Part model, mm, in its own coordinate system. Face numbers are marked on the shaded views. A direction names the side the tool comes from. Give positions to 0.01 mm unless a question says otherwise; leave off trailing zeros. Write each loop counter-clockwise with the first axis right and the second up, starting at its lowest first coordinate (ties: lowest second). Pieces come first, ordered by that corner, then holes.
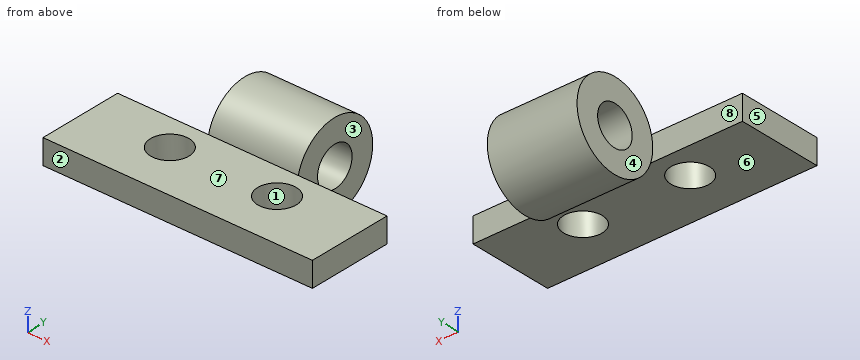
from build123d import *

# Parameters (mm, degrees)
SKETCH1_W           = 24.892
SKETCH1_H           = 7.874
BOSS_EXTRUDE1_DEPTH = 2.286
SKETCH4_R           = 4
BOSS_EXTRUDE3_DEPTH = 16.58
SKETCH5_R           = 1.825
CUT_EXTRUDE2_DEPTH  = 16.58
CUT_EXTRUDE3_DEPTH  = 8.29
SKETCH8_R           = 1.778
CUT_EXTRUDE4_DEPTH  = 8.29
SKETCH9_W           = 2.190957137
SKETCH9_H           = 1.309901185
SKETCH9_W_2         = 1.781735984
SKETCH9_H_2         = 0.803323297
CUT_EXTRUDE5_DEPTH  = 8.29


with BuildPart() as part:
    # Sketch1 → Boss-Extrude1 (new body)
    with BuildSketch(Plane.XY):
        with Locations((-11.83196875, 3.65678125)):
            Rectangle(SKETCH1_W, SKETCH1_H)
    extrude(amount=BOSS_EXTRUDE1_DEPTH)

    # Sketch4 → Boss-Extrude3 (add)
    with BuildSketch(Plane.ZY.offset(24.27796875)):
        with Locations((1.143, 11.58378125)):
            Circle(SKETCH4_R)
    extrude(amount=-BOSS_EXTRUDE3_DEPTH)

    # Sketch5 → Cut-Extrude2 (cut)
    with BuildSketch(Plane.ZY.offset(24.27796875)):
        with Locations((1.143, 11.58378125)):
            Circle(SKETCH5_R)
    extrude(amount=-CUT_EXTRUDE2_DEPTH, mode=Mode.SUBTRACT)

    # Sketch7 → Cut-Extrude3 (cut)
    with BuildSketch(Plane.ZY.offset(24.27796875)):
        Polygon((0.43016706, 7.59378125), (-5.580589686, 7.59378125), (-5.580589686, 19.623956734), (9.570834238, 19.623956734), (9.570834238, 7.59378125), align=None)
    extrude(amount=-CUT_EXTRUDE3_DEPTH, mode=Mode.SUBTRACT)

    # Sketch8 → Cut-Extrude4 (cut)
    with BuildSketch(Plane(origin=(0, 0, 0), x_dir=(-1, 0, 0), z_dir=(0, 0, -1))):
        with Locations((6.87896875, 4.54578125)):
            Circle(SKETCH8_R)
        with Locations((16.78496875, 4.54578125)):
            Circle(SKETCH8_R)
    extrude(amount=-CUT_EXTRUDE4_DEPTH, mode=Mode.SUBTRACT)

    # Sketch9 → Cut-Extrude5 (cut)
    with BuildSketch(Plane.ZY.offset(24.27796875)):
        with Locations((3.381478569, 7.915515048)):
            Rectangle(SKETCH9_W, SKETCH9_H)
        with Locations((-0.890867992, 7.662226104)):
            Rectangle(SKETCH9_W_2, SKETCH9_H_2)
    extrude(amount=-CUT_EXTRUDE5_DEPTH, mode=Mode.SUBTRACT)


solid = part.part
1) 3-axis set-ups, long thin cutter, end or side, ignore diameter. For the marked faces 4, 5, 6, 7 and 8: which of +Z, -Z, +X, -X, +Y, -Y reach the whole face in a straight line?
Check result:
face 4: +Z, -Z, -X, +Y
face 5: +Z, -Z, -X, +Y, -Y
face 6: -Z, +X, -X, -Y
face 7: +Z, +X, -X, -Y
face 8: none
2) Saw through at D-D (y = 2). Write the cut outline in (x, z), and give its area (3 significant figures).
Check result:
outline: (-24.28, 0) - (0.61, 0) - (0.61, 2.29) - (-24.28, 2.29) - close
area: 56.9 mm2
3) Flat gauge pins, fed straight in: P1, Ø2, axis at x = -14, y = 5.5, coming from the +Z side; P2, Ø1.5, axis at x = -16, y = 8.5, coming from the +Z side; P3, Ø1.5, axis at x = -13.5, z = 0, coming from the +Y side; P4, Ø2, axis at x = -16.78, y = 4.55, coming from the -Z side. Where does each tip first touch, or does it go through?
Check result:
P1: stops at z = 2.29
P2: stops at z = 4.39
P3: stops at y = 15.56
P4: passes through
4) Drill centre lines: L1, parallel to Y at x = -20.5, z = 2; L2, parallel to X at y = 14.25, z = 3; L3, parallel to X at y = 3.5, z = 0.75. Where is each one in solid material? Low to high.
Check result:
L1: y = -0.28 to 7.59
L2: x = -15.99 to -7.7
L3: x = -24.28 to -18.22, -15.35 to -8.32, -5.44 to 0.61
5) Saw through at A-A (z = 1.75). Write the cut outline in (x, y), and give its area (3 significant figures).
Check result:
outline: (-24.28, -0.28) - (0.61, -0.28) - (0.61, 7.59) - (-24.28, 7.59) - close; (-15.99, 7.63) - (-7.7, 7.63) - (-7.7, 9.86) - (-15.99, 9.86) - close; (-15.99, 13.3) - (-7.7, 13.3) - (-7.7, 15.54) - (-15.99, 15.54) - close; hole circle Ø3.56 at (-16.78, 4.55); hole circle Ø3.56 at (-6.88, 4.55)
area: 213 mm2
6) Saw through at B-B (x = -12). Write the cut outline in (y, z) (3 decimals), and give its area (3 significant figures).
Check result:
outline: (-0.28, 0) - (7.594, 0) - (7.594, 0.86) arc R4 ccw (long way) to (7.594, 1.426) - (7.594, 2.286) - (-0.28, 2.286) - close; hole circle Ø3.65 at (11.584, 1.143)
area: 57.8 mm2
7) Saw through at C-C (x = -6). Write the cut outline in (y, z), and give its area (3 significant figures).
Check result:
outline: (-0.28, 0) - (3, 0) - (3, 2.29) - (-0.28, 2.29) - close; (6.09, 0) - (7.59, 0) - (7.59, 2.29) - (6.09, 2.29) - close
area: 10.9 mm2
8) Mould opens along Y. For the marked faces 1, 2 and 3 say: +Y half, -Y half, draft (parallel to the pull), parting line (faces both ways), or undercut.
Check result:
face 1: undercut
face 2: -Y half
face 3: draft
